For this review, take the finished solid that the model builds, in its own axes (mm). A direction names the side the tool comes from. Coordinates: 2 decimals unless noted, no trailing zeros. Loops run counter-clockwise (first coordinate to the right, second up) from the corner with the lowest first, then second, coordinate; pieces in that order, holes last. Notation, with made-up numbers: (-27, -14) - (29, -14) arc R18 cw to (29, 10) - close; hole circle Ø3 at (28.5, 27.5). An arc over 180 degrees is marked (long way). Use one line per item in the form item = value. Start each with the question number.
1. Add section D-D on z = -9. Give the boundary of the cut face in (x, y), and give its area (3 significant figures).
2. Add section C-C on y = 35. Give the boundary of the cut face in (x, z), and give its area (3 significant figures).
3. Add section B-B on x = -929. Give the boundary of the cut face in (y, z).
4. Add section A-A on y = 83. Give the boundary of the cut face in (x, z), and give its area (3 significant figures).
5. For pin 1 Ø1.2 at (x, z) = (-1002, -32.5) entering from +Y; pin 2 Ø2.5 at (y, z) = (84.5, -35.5) entering from +X; pin 3 Ø20 at (x, y) = (-978.5, 97) entering from +Z, all flat-tipped, find the tip position at first contact; note any pin that passes through.
6. Machinability: for faces 4 (the face through (-880.665, 88, 5)), 5 (the face through (-899, 100, -37.098)), 6 (the face through (-1003.06, 48.44, 8.85)), which of the approach directions +Z, -Z, +X, -X, +Y, -Y give a long, thin tool a straight path to every point of the face, cutting with its end or side? Answer none if there is none.
7. Draft analysis for pull direction Z (two halves, no side actions). For faces 1 (the face through (-994.423, 46.166, -40.507)), 2 (the face through (-909, 101.7, -35)), 3 (the face through (-980, 100, 6.381)), state which applies: +Z half, -Z half, draft (parallel to the pull), parting line (faces both ways), or undercut.
8. To check wall thickness, follow probe 1 along Z at (x, y) = (-979, 43.5); probe 2 along X at (y, z) = (29.5, -36.5); probe 3 along Y at (x, z) = (-973, -17). State the ranges of each line that lie inside material, in increasing order.
```python
from build123d import *

# Parameters (mm, degrees)
SKETCH1_W             = 142
SKETCH1_H             = 47
BOSS_EXTRUDE1_DEPTH   = 110
SKETCH2_W             = 42
SKETCH2_H             = 49.6
CUT_EXTRUDE1_DEPTH    = 137
SKETCH4_W             = 33.598594883
SKETCH4_H             = 47
CUT_EXTRUDE3_DEPTH    = 10
CUT_EXTRUDE9_DEPTH    = 184.776508378
SKETCH8_W             = 12
SKETCH8_H             = 39.032308198
SKETCH8_W_2           = 45
CUT_EXTRUDE12_DEPTH   = 1018.719156625
SKETCH11_R            = 2.5
CUT_EXTRUDE13_DEPTH   = 1018.639266937
FILLET5_R             = 5
SKETCH13_W            = 47
SKETCH13_H            = 52.1
CUT_EXTRUDE14_DEPTH   = 91.7220084
BOSS_EXTRUDE2_DEPTH   = 50.2779916
BOSS_EXTRUDE3_DEPTH   = 50.2779916
SKETCH17_W            = 42
SKETCH17_H            = 49.6
CUT_EXTRUDE15_DEPTH   = 182.086628796
M6_TAPPED_HOLE1_D     = 5
M6_TAPPED_HOLE1_DEPTH = 15
M6_TAPPED_HOLE1_TIP   = 1.502151548


with BuildPart() as part:
    # Sketch1 → Boss-Extrude1 (new body)
    with BuildSketch(Plane(origin=(0, 0, 0), x_dir=(1, 0, 0), z_dir=(0, 1, 0))):
        with Locations((-939.664772198, 15.356209692)):
            Rectangle(SKETCH1_W, SKETCH1_H)
    extrude(amount=BOSS_EXTRUDE1_DEPTH)

    # Sketch2 → Cut-Extrude1 (cut)
    with BuildSketch(Plane(origin=(-868.664772198, 0, 0), x_dir=(0, 0, -1), z_dir=(1, 0, 0))):
        with Locations((15.356209692, 27.3)):
            Rectangle(SKETCH2_W, SKETCH2_H)
    extrude(amount=-CUT_EXTRUDE1_DEPTH, mode=Mode.SUBTRACT)

    # Sketch4 → Cut-Extrude3 (cut)
    with BuildSketch(Plane.XZ):
        with Locations((-943.587483157, -15.356209692)):
            Rectangle(SKETCH4_W, SKETCH4_H)
    extrude(amount=-CUT_EXTRUDE3_DEPTH, mode=Mode.SUBTRACT)

    # Sketch5 → Cut-Extrude9 (cut, through all)
    with BuildSketch(Plane(origin=(-868.664772198, 0, 0), x_dir=(0, 0, -1), z_dir=(1, 0, 0))):
        with BuildLine():
            Line((32.925507135, 110), (-2.21308775, 110))
            Line((-2.21308775, 110), (-2.21308775, 91.687910414))
            ThreePointArc((-2.21308775, 91.687910414), (15.356209692, 63.4), (32.925507135, 91.687910414))
            Line((32.925507135, 91.687910414), (32.925507135, 110))
        make_face()
        with BuildLine():
            Line((-6.380897296, 90.501069346), (-6.380897296, 110))
            Line((-6.380897296, 110), (-8.143790308, 110))
            Line((-8.143790308, 110), (-8.143790308, 56))
            Line((-8.143790308, 56), (-4.23948935, 70.967691802))
            ThreePointArc((-4.23948935, 70.967691802), (-7.501795977, 80.49411924), (-6.380897296, 90.501069346))
        make_face()
        with BuildLine():
            ThreePointArc((37.098087644, 90.487229439), (38.21341655, 80.486843377), (34.951908735, 70.967691802))
            Line((34.951908735, 70.967691802), (38.856209692, 56))
            Line((38.856209692, 56), (38.856209692, 110))
            Line((38.856209692, 110), (37.098087644, 110))
            Line((37.098087644, 110), (37.098087644, 90.487229439))
        make_face()
    extrude(amount=-CUT_EXTRUDE9_DEPTH, mode=Mode.SUBTRACT)

    # Sketch8 → Cut-Extrude12 (cut, through all)
    with BuildSketch(Plane.XY.offset(8.143790308)):
        with Locations((-1004.664772198, 90.483845901)):
            Rectangle(SKETCH8_W, SKETCH8_H)
        with Locations((-939.664772198, 90.483845901)):
            Rectangle(SKETCH8_W_2, SKETCH8_H)
        with Locations((-874.664772198, 90.483845901)):
            Rectangle(SKETCH8_W, SKETCH8_H)
    extrude(amount=-CUT_EXTRUDE12_DEPTH, mode=Mode.SUBTRACT)

    # Sketch11 → Cut-Extrude13 (cut, through all)
    with BuildSketch(Plane.XY.offset(6.380897296)):
        with Locations((-988.664772198, 100)):
            Circle(SKETCH11_R)
        with Locations((-972.164772198, 100)):
            Circle(SKETCH11_R)
        with Locations((-907.164772198, 100)):
            Circle(SKETCH11_R)
        with Locations((-890.664772198, 100)):
            Circle(SKETCH11_R)
    extrude(amount=-CUT_EXTRUDE13_DEPTH, mode=Mode.SUBTRACT)

    # Fillet5
    fillet5_edges = [part.edges().sort_by_distance(p)[0] for p in [
        (-998.664772198, 110, 4.296992523),
        (-998.664772198, 110, -35.01179739),
        (-917.164772198, 110, 4.296992523),
        (-962.164772198, 110, 4.296992523),
        (-962.164772198, 110, -35.01179739),
        (-917.164772198, 110, -35.01179739),
        (-880.664772198, 110, 4.296992523),
        (-880.664772198, 110, -35.01179739),
    ]]
    fillet(fillet5_edges, radius=FILLET5_R)

    # Sketch13 → Cut-Extrude14 (cut)
    with BuildSketch(Plane(origin=(-868.664772198, 0, 0), x_dir=(0, 0, -1), z_dir=(1, 0, 0))):
        with Locations((15.356209692, 26.05)):
            Rectangle(SKETCH13_W, SKETCH13_H)
    extrude(amount=-CUT_EXTRUDE14_DEPTH, mode=Mode.SUBTRACT)

    # Sketch15 → Boss-Extrude2 (add)
    with BuildSketch(Plane(origin=(-960.386780598, 0, 0), x_dir=(0, 0, -1), z_dir=(1, 0, 0))):
        Polygon((-8.143790308, 52.1), (-13.143790308, 52.1), (-13.143790308, -5), (43.856209692, -5), (43.856209692, 52.1), (38.856209692, 52.1), (38.856209692, 0), (-8.143790308, 0), align=None)
    extrude(amount=-BOSS_EXTRUDE2_DEPTH)

    # Sketch16 → Boss-Extrude3 (add)
    with BuildSketch(Plane.ZY.offset(1010.664772198)):
        Polygon((-38.856209692, 56), (-43.856209692, 52.1), (-38.856209692, 52.1), align=None)
        Polygon((8.143790308, 56), (13.143790308, 52.1), (8.143790308, 52.1), align=None)
    extrude(amount=-BOSS_EXTRUDE3_DEPTH)

    # Sketch17 → Cut-Extrude15 (cut, through all)
    with BuildSketch(Plane(origin=(-1005.664772198, 0, 0), x_dir=(0, 0, -1), z_dir=(1, 0, 0))):
        with Locations((15.356209692, 27.3)):
            Rectangle(SKETCH17_W, SKETCH17_H)
    extrude(amount=-CUT_EXTRUDE15_DEPTH, mode=Mode.SUBTRACT)

    # M6 Tapped Hole1
    with Locations(Plane(origin=(-1010.664772198, 46, -40.106209692), x_dir=(0, 0, -1), z_dir=(-1, 0, 0))):
        with Locations((0, 0), (0, 45), (-49.5, 45), (-49.5, 0)):
            Hole(M6_TAPPED_HOLE1_D / 2, depth=M6_TAPPED_HOLE1_DEPTH)
            with Locations((0, 0, -(M6_TAPPED_HOLE1_DEPTH + M6_TAPPED_HOLE1_TIP / 2))):  # 118° drill point
                Cone(0, M6_TAPPED_HOLE1_D / 2, M6_TAPPED_HOLE1_TIP, mode=Mode.SUBTRACT)


solid = part.part
```
Conclusion:
q1.outline = (-1010.66, -5) - (-960.39, -5) - (-960.39, 2.5) - (-1010.66, 2.5) - close; (-1010.66, 52.1) - (-868.66, 52.1) - (-868.66, 64.46) - (-1010.66, 64.46) - close
q1.area = 2,130 mm^2
q2.outline = (-1010.66, -43.86) - (-960.39, -43.86) - (-960.39, -36.36) - (-1010.66, -36.36) - close; (-1010.66, 5.64) - (-960.39, 5.64) - (-960.39, 13.14) - (-1010.66, 13.14) - close
q2.area = 754 mm^2
q3.outline = (52.1, -38.86) - (56, -38.86) - (70.97, -34.95) - (70.97, -30.83) arc R19.6 cw to (70.97, 0.12) - (70.97, 4.24) - (56, 8.14) - (52.1, 8.14) - close
q4.outline = (-998.66, -38.35) - (-962.16, -38.35) - (-962.16, -34.96) - (-998.66, -34.96) - close; (-998.66, 4.24) - (-962.16, 4.24) - (-962.16, 7.64) - (-998.66, 7.64) - close; (-917.16, -38.35) - (-880.66, -38.35) - (-880.66, -34.96) - (-917.16, -34.96) - close; (-917.16, 4.24) - (-880.66, 4.24) - (-880.66, 7.64) - (-917.16, 7.64) - close
q4.area = 496 mm^2
q5.pin_1 = 70.97
q5.pin_2 = -880.66
q5.pin_3 = 7.29
q6.face_4 = +Z, -Z, +X, +Y
q6.face_5 = -Z, +X, -X, +Y
q6.face_6 = -X
q7.face_1 = undercut
q7.face_2 = draft
q7.face_3 = +Z half
q8.probe_1 = -43.86 to -36.36, 5.64 to 13.14
q8.probe_2 = -1010.66 to -960.39
q8.probe_3 = -5 to 2.5, 52.1 to 63.47
